Can you work these out from the model? Positions are in its coordinate system, mm. Give positions to 0.01 mm unless a question says otherwise; leave off trailing zeros. Write each question's results on one line, items separated by ' | '.
from build123d import *

# Parameters (mm, degrees)
F0_W     = 285
F0_H     = 20
F1_DEPTH = 5
F2_R     = 9.99999
F3_R     = 5
F3_R_2   = 5.4133078472
F4_DEPTH = 20


# Not quite as in the source:
# - a fillet or chamfer is up to 0.001 mm smaller than in the source, because OpenCascade refuses the exact size


with BuildPart() as f1:
    # F0 (on Front) → F1 (new body)
    with BuildSketch(Plane.XZ):
        with Locations((-142.5, 10)):
            Rectangle(F0_W, F0_H)
    extrude(amount=F1_DEPTH)

    # F2 (radius 10 in the source; OpenCascade refuses exactly that, so slightly less here)
    f2_edges = [f1.edges().sort_by_distance(p)[0] for p in [
        (0, -2.5, 20),
        (0, -2.5, 0),
        (-285, -2.5, 20),
        (-285, -2.5, 0),
    ]]
    fillet(f2_edges, radius=F2_R)

    # F3 (on Front) → F4 (cut)
    with BuildSketch(Plane.XZ):
        with Locations((-274.8824357986, 10.0639369339)):
            Circle(F3_R)
        with Locations((-9.8824357986, 10.070726499)):
            Circle(F3_R_2)
    extrude(amount=F4_DEPTH, mode=Mode.SUBTRACT)


solid = f1.part
(1) I need wall thicknesses on L1, parallel to X at y = -1.65, z = 9.5; L2, parallel to X at y = -0.25, z = 8.75; L3, parallel to X at y = -3.2, z = 3.5. Which ranges of each line are inside material? Lowest first, please. Write a range as from..to.
Data:
L1: x = -284.99..-279.85, -269.91..-15.27, -4.5..-0.01 | L2: x = -284.92..-279.71, -270.06..-15.13, -4.63..-0.08 | L3: x = -282.6..-2.4
(2) We'd pull the mould along Z, two halves only. Please class faces 1 (the face through (-144, 0, 10)), 2 (the face through (-144, -2, 20)), 3 (the face through (-13.9, -2.5, 13.7)): +Z half, -Z half, draft (parallel to the pull), parting line (faces both ways), or undercut.
Data:
face 1: draft | face 2: +Z half | face 3: undercut
(3) Imagine slicing it at A-A, the plane y = -2.3. Count the separate pieces of the cut face and the enclosed holes in it, plus the area to 3 significant figures.
Data:
separate pieces: 1 | enclosed holes: 2 | area: 5,440 mm2
(4) Will this pin go through, and if not, where does the flat tip stop? P1, Ø3, axis at y = -4.5, z = 3, coming from the -X side.
Data:
P1: stops at x = -283.35
